Work out the finished part from the listing and answer in its coordinate system (mm). A direction names the side the tool comes from. Coordinates: 2 decimals unless noted, no trailing zeros. Loops run counter-clockwise (first coordinate to the right, second up) from the corner with the lowest first, then second, coordinate; pieces in that order, holes last. Notation, with made-up numbers: (15.5, -13) -> (39.5, -13) arc R18 cw to (39.5, 2) -> close; hole circle Ø4 at (12, -15). An arc over 180 degrees is marked (long way). Answer as CSV lines item,"result".
```python
from build123d import *

# Parameters (mm, degrees)
CYLINDER099_R     = 29
CYLINDER099_DEPTH = 46
CYLINDER097_R     = 28
CYLINDER097_DEPTH = 30
CYLINDER098_R     = 30
CYLINDER098_DEPTH = 30
CYLINDER095_R     = 25
CYLINDER095_DEPTH = 10
CYLINDER096_R     = 28
CYLINDER096_DEPTH = 10


with BuildPart() as cylinder099:
    # Cylinder099 → Cylinder099 (new body)
    with BuildSketch(Plane(origin=(0, 0, 41), x_dir=(1, 0, 0), z_dir=(0, -1, 0))):
        Circle(CYLINDER099_R)
    extrude(amount=CYLINDER099_DEPTH)


with BuildPart() as cylinder097:
    # Cylinder097 → Cylinder097 (new body)
    with BuildSketch(Plane.XY.offset(-10)):
        Circle(CYLINDER097_R)
    extrude(amount=CYLINDER097_DEPTH)


with BuildPart() as cut103:
    # Cylinder098 → Cylinder098 (new body)
    with BuildSketch(Plane.XY.offset(-10)):
        Circle(CYLINDER098_R)
    extrude(amount=CYLINDER098_DEPTH)

    # Cut103: cut Cylinder097
    add(cylinder097.part, mode=Mode.SUBTRACT)


with BuildPart() as cylinder095:
    # Cylinder095 → Cylinder095 (new body)
    with BuildSketch(Plane.XY):
        Circle(CYLINDER095_R)
    extrude(amount=CYLINDER095_DEPTH)


with BuildPart() as cut104:
    # Cylinder096 → Cylinder096 (new body)
    with BuildSketch(Plane.XY):
        Circle(CYLINDER096_R)
    extrude(amount=CYLINDER096_DEPTH)

    # Cut102: cut Cylinder095
    add(cylinder095.part, mode=Mode.SUBTRACT)

    # Fusion029: union Cut103
    add(cut103.part)

    # Cut104: cut Cylinder099
    add(cylinder099.part, mode=Mode.SUBTRACT)


solid = cut104.part
```
(1) A cutting plane is placed at B-B, the plane x = 0. Write down the section's boundary in (y, z), and give its area (3 significant figures).
Computed values:
outline,"(-30, -10) -> (-28, -10) -> (-28, 0) -> (-25, 0) -> (-25, 10) -> (-28, 10) -> (-28, 12) -> (-30, 12) -> close; (25, 0) -> (28, 0) -> (28, -10) -> (30, -10) -> (30, 20) -> (28, 20) -> (28, 10) -> (25, 10) -> close"
area,"164 mm2"
(2) Flat-ended cylindrical pins translate along their axes: pin 1 Ø1 at (x, z) = (23, 15.5) entering from -Y; pin 2 Ø10 at (x, z) = (14.5, -1.5) entering from -Y; pin 3 Ø12 at (x, z) = (12, 11) entering from -Y. Find the tip coordinate at first contact, or state that the pin passes through.
Computed values:
pin 1,"y = -19.84"
pin 2,"y = -28.46"
pin 3,"y = -29.39"
(3) Which of the six approach directions +Z, -Z, +X, -X, +Y, -Y give full straight-line access (tool end or side, diameter ignored) to faces 5 (the face through (25.865, -10.724, -5.07)), 6 (the face through (-3.65, 27.76, 14.93)), 7 (the face through (-25, 13, -10))?
Computed values:
face 5,"-Z"
face 6,"+Z"
face 7,"-Z, +X, -X, +Y, -Y"
(4) A cutting plane is placed at C-C, the plane z = -7.5. Write down the section's boundary in (x, y), and give its area (3 significant figures).
Computed values:
outline,"circle Ø60 at (0, 0); hole circle Ø56 at (0, 0)"
area,"364 mm2"
(5) Consider line 1 along Y through (x, z) = (0, 5.5); line 2 along X through (y, z) = (0, 14); line 3 along Y through (x, z) = (-3, 1). Determine where each line is inside the solid, lowest interval first.
Computed values:
line 1,"-30 to -25, 25 to 30"
line 2,"-30 to -28, 28 to 30"
line 3,"-29.85 to -24.82, 24.82 to 29.85"
(6) For a pull along X with two mould halves and no side action, classify faces 1 (the face through (-3.905, 29.745, 4.79)), 2 (the face through (9, 27, 20)), 3 (the face through (23.846, 7.509, 4.93)), 4 (the face through (-0.1, -28.2, 12)) as pulls with the +X half, pulls with the -X half, needs draft (parallel to the pull), parting line crosses it, or undercut.
Computed values:
face 1,"parting line crosses it"
face 2,"needs draft"
face 3,"undercut"
face 4,"undercut"
(7) A cutting plane is placed at A-A, the plane y = 0. Write down the section's boundary in (x, z), and give its area (3 significant figures).
Computed values:
outline,"(-30, -10) -> (-28, -10) -> (-28, 0) -> (-25, 0) -> (-25, 10) -> (-28, 10) -> (-28, 20) -> (-30, 20) -> close; (25, 0) -> (28, 0) -> (28, -10) -> (30, -10) -> (30, 20) -> (28, 20) -> (28, 10) -> (25, 10) -> close"
area,"180 mm2"
(8) A cutting plane is placed at D-D, the plane z = 18. Write down the section's boundary in (x, y).
Computed values:
outline,"(-17.66, -24.25) -> (-17.66, -21.73) arc R28 cw (long way) to (17.66, -21.73) -> (17.66, -24.25) arc R30 ccw (long way) to start"
